Autodesk Inventor part; units mm, degrees
ref_plane "YZ Plane" through (0, 0, 0) normal (1, 0, 0) x (0, 1, 0)
ref_plane "XZ Plane" through (0, 0, 0) normal (0, 1, 0) x (-1, 0, 0)
ref_plane "XY Plane" through (0, 0, 0) normal (0, 0, 1) x (1, 0, 0)
sketch "Sketch1" plane through (0, 0, 0) normal (0, 1, 0) x (-1, 0, 0)
  line L0 (7.5264, 21.8341) -> (7.5264, 13.5841)
  line L1 (7.5264, 13.5841) -> (1.6928, 7.7505)
  line L2 (1.6928, 7.7505) -> (-6.5572, 7.7505)
  line L3 (7.5264, 21.8341) -> (1.6928, 27.6678)
  line L4 (1.6928, 27.6678) -> (-6.5572, 27.6678)
  line L5 (-6.5572, 27.6678) -> (-12.3908, 21.8341)
  line L6 (-12.3908, 21.8341) -> (-12.3908, 13.5841)
  line L7 (-12.3908, 13.5841) -> (-6.5572, 7.7505)
  line L8 (8.5264, 22.2483) -> (8.5264, 13.1699)
  line L9 (8.5264, 13.1699) -> (2.107, 6.7505)
  line L10 (2.107, 6.7505) -> (-6.9714, 6.7505)
  line L11 (8.5264, 22.2483) -> (2.107, 28.6678)
  line L12 (2.107, 28.6678) -> (-6.9714, 28.6678)
  line L13 (-6.9714, 28.6678) -> (-13.3908, 22.2483)
  line L14 (-13.3908, 22.2483) -> (-13.3908, 13.1699)
  line L15 (-13.3908, 13.1699) -> (-6.9714, 6.7505)
  point P0 (0, 0)
  point P1 (1, 1)
  dimension "d0" = 8.25
  dimension "d3" = 8.25
  dimension "d5" = 8.25
  dimension "d7" = 8.25
  dimension "d8" = 8.25
  dimension "d9" = 8.25
  dimension "d12" = 8.25
  dimension "d17" = 8.25
  dimension "d29" = 1
  dimension "d31" = 1
  dimension "d32" = 1
  dimension "d33" = 1
  dimension "d101" = 135
  dimension "d102" = 135
  dimension "d115" = 135
  dimension "d116" = 135
  dimension "d135" = 1
  dimension "d138" = 1
  dimension "d139" = 135
  dimension "d140" = 135
  dimension "d141" = 135
  dimension "d142" = 135
  dimension "d143" = 1
  dimension "d144" = 1
  dimension "d145" = 135
  dimension "d146" = 135
  dimension "d147" = 135
  dimension "d148" = 135
  dimension "d149" = 135
  dimension "d150" = 135
  dimension "d151" = 135
  dimension "d152" = 135
extrude "OutsideHeight" add sketch "Sketch1" along normal blind 10
extrude "BaseHeight" add sketch "Sketch1" along normal blind 1 contours L0 L1 L2 L7 L6 L5 L4 L3
sketch "Sketch5" plane through (0, 1, 0) normal (0, 1, 0) x (1, 0, 0)
  line L0 (-1.6928, -27.6678) -> (-7.5264, -21.8341)
  line L1 (-7.5264, -13.5841) -> (-1.6928, -7.7505)
  line L2 (-7.5264, -21.8341) -> (-7.5264, -13.5841)
  line L3 (-7.5264, -13.5841) -> (-1.6928, -7.7505)
  line L4 (-1.6928, -7.7505) -> (6.5572, -7.7505)
  line L5 (-1.6928, -7.7505) -> (6.5572, -7.7505)
  line L6 (6.5572, -7.7505) -> (12.3908, -13.5841)
  line L7 (12.3908, -13.5841) -> (12.7122, -18.5063)
  line L8 (12.3908, -13.5841) -> (12.3908, -21.8341)
  line L9 (12.3908, -13.5841) -> (12.3908, -21.8341)
  line L10 (12.3908, -21.8341) -> (6.5572, -27.6678)
  line L11 (6.5572, -27.6678) -> (-1.6928, -27.6678)
  line L12 (-1.6928, -27.6678) -> (-7.5264, -21.8341)
  line L13 (-5.5264, -21.0057) -> (-5.5264, -14.4125)
  line L14 (-5.5264, -14.4125) -> (-0.8644, -9.7505)
  line L15 (-0.8644, -9.7505) -> (5.7288, -9.7505)
  line L16 (5.7288, -9.7505) -> (10.3908, -14.4125)
  line L17 (10.3908, -14.4125) -> (10.3908, -21.0057)
  line L18 (10.3908, -21.0057) -> (5.7288, -25.6678)
  line L19 (5.7288, -25.6678) -> (-0.8644, -25.6678)
  line L20 (-0.8644, -25.6678) -> (-5.5264, -21.0057)
  point P0 (0, 0)
  point P1 (-1.6932, -27.6674)
  dimension "d94" = 135
  dimension "d95" = 135
  dimension "d125" = 135
  dimension "d126" = 135
  dimension "d127" = 135
  dimension "d128" = 135
  dimension "d129" = 135
  dimension "d130" = 135
  dimension "d131" = 2
extrude "BaseCut" cut sketch "Sketch5" against normal blind 1 contours L13 L14 L15 L16 L17 L18 L19 L20
equation "\"d3\" = d0"
equation "\"d5\" = d0"
equation "\"d7\" = d0"
equation "\"d8\" = d0"
equation "\"d9\" = d0"
equation "\"d12\" = d0"
equation "\"d17\" = d0"
equation "\"d115\" = d110"
equation "\"d57\" = d72"
equation "\"d66\" = d57"
properties part number "_3DPrint"
Could you check a few things on this model? Use its own coordinates, in mm. A direction names the side the tool comes from. Give positions to 0.01 mm unless a question says otherwise; leave off trailing zeros. Order: outer loops, then holes, each group sorted by start corner. A loop starts at its lowest first (then second) coordinate and runs counter-clockwise, first axis right, second up. Notation, with made-up numbers: (35, -18.75) - (69, -18.75) arc R13 ccw to (69, 0.25) - close; hole circle Ø8 at (24, 52.25). An arc over 180 degrees is marked (long way). Return JSON: item names as keys, results as strings. Group by question number.
Q1. Thinking about a two-plate mould opening in Z: for faces 4 (the face through (2, 5, 6.75)), 5 (the face through (2, 5, 28.668)), 6 (the face through (2.4, 0.5, 9.75)), which applies, pulls with the +Z half, pulls with the -Z half, needs draft (parallel to the pull), parting line crosses it, or undercut?
Q2. Suppose I cut it at A-A, the plane x = 1.25. Please give me the cut outline in (y, z), and give its area (3 significant figures).
Q3. Suppose I cut it at B-B, the plane y = 3.5. Please give me the cut outline in (x, z).
Q4. Which directions (+Z, -Z, +X, -X, +Y, -Y) give clear straight access to the entire face, cutting with the end or side of a thin tool? Please do faces 1 (the face through (-5, 0, 23)), 2 (the face through (2, 5, 27.668)), 3 (the face through (2.5, 0.5, 25.668)).
Q5. Suppose I cut it at D-D, the plane z = 26.75. Please give me the cut outline in (x, y), and give its area (3 significant figures).
Q6. Will these pins go through, and if not, where does the flat tip stop? pin 1 Ø1 at (y, z) = (6.5, 11) entering from -X; pin 2 Ø5 at (x, z) = (-3, 13.5) entering from +Y; pin 3 Ø5 at (x, z) = (5, 20) entering from +Y.
Q7. Please list where these lines run through material, in increasing order: line 1 along Z through (x, y) = (6, 3.5); line 2 along X through (y, z) = (6.5, 13.75); line 3 along Y through (x, z) = (11.75, 20). Write a range as [from, to].
Q8. Suppose I cut it at C-C, the plane z = 24. Please give me the cut outline in (x, y).
Resolved:
{
 "1": {"face 4": "pulls with the -Z half", "face 5": "pulls with the +Z half", "face 6": "undercut"},
 "2": {"outline": "(0, 6.75) - (10, 6.75) - (10, 7.75) - (1, 7.75) - (1, 9.75) - (0, 9.75) - close; (0, 25.67) - (1, 25.67) - (1, 27.67) - (10, 27.67) - (10, 28.67) - (0, 28.67) - close", "area": "24.0 mm2"},
 "3": {"outline": "(-8.53, 13.17) - (-2.11, 6.75) - (6.97, 6.75) - (13.39, 13.17) - (13.39, 22.25) - (6.97, 28.67) - (-2.11, 28.67) - (-8.53, 22.25) - close; hole (-7.53, 13.58) - (-1.69, 7.75) - (6.56, 7.75) - (12.39, 13.58) - (12.39, 21.83) - (6.56, 27.67) - (-1.69, 27.67) - (-7.53, 21.83) - close"},
 "4": {"face 1": "+Z, -Z, +X, -X, -Y", "face 2": "+Y", "face 3": "+Y, -Y"},
 "5": {"outline": "(-4.02, 0) - (8.89, 0) - (8.89, 10) - (7.47, 10) - (7.47, 1) - (-2.61, 1) - (-2.61, 10) - (-4.02, 10) - close", "area": "38.4 mm2"},
 "6": {"pin 1": "stops at x = -6.86", "pin 2": "stops at y = 1", "pin 3": "passes through"},
 "7": {"line 1": "z = [6.75, 7.75], [27.67, 28.67]", "line 2": "x = [-8.53, -7.53], [12.39, 13.39]", "line 3": "y = [0, 1]"},
 "8": {"outline": "(-6.77, 0) - (-2.53, 0) - (-2.53, 1) - (-5.36, 1) - (-5.36, 10) - (-6.77, 10) - close; (7.4, 0) - (11.64, 0) - (11.64, 10) - (10.22, 10) - (10.22, 1) - (7.4, 1) - close"}
}
